Check sheet for the modelled part. Datum: model origin and axes. Units: mm. Face numbers are marked on the shaded views. A direction names the side the tool comes from. Round coordinates to 2 decimals unless told otherwise and drop trailing zeros. Order: outer loops, then holes, each group sorted by start corner. A loop starts at its lowest first (then second) coordinate and runs counter-clockwise, first axis right, second up. Notation, with made-up numbers: (80, -40) -> (90, -40) arc R13 cw to (90, -28) -> close; hole circle Ø4 at (61.5, 51). An arc over 180 degrees is marked (long way). Answer in a Markdown table with one row per item.
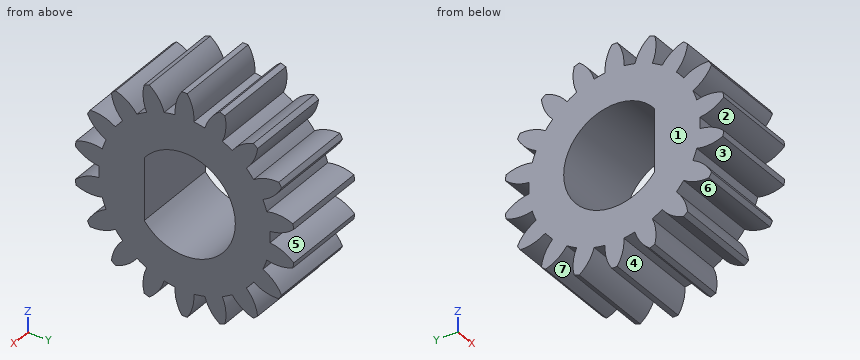
from build123d import *

# Parameters (mm, degrees)
BASPROSKE_W     = 4
BASPROSKE_H     = 5
TOOTHCUT_DEPTH  = 9.124038405
TEETHCUTS_COUNT = 18
TEETHCUTS_ANGLE = 340
BORE_DEPTH      = 50.0000508


with BuildPart() as part:
    # BasProSke → Base-Revolve (revolve)
    with BuildSketch(Plane(origin=(0, 0, 0), x_dir=(1, 0, 0), z_dir=(0, 1, 0)), mode=Mode.PRIVATE) as base_revolve_sk:
        with Locations((2, 2.5)):
            Rectangle(BASPROSKE_W, BASPROSKE_H)
    revolve(base_revolve_sk.sketch.rotate(Axis((-10, 0, 0), (1, 0, 0)), 180), axis=Axis((-10, 0, 0), (1, 0, 0)))

    # TooCutSke → ToothCut (cut, through all)
    with BuildSketch(Plane(origin=(0, 0, 0), x_dir=(0, 0, -1), z_dir=(1, 0, 0))):
        with BuildLine():
            ThreePointArc((0.25527463, 3.865580275), (0, 3.874), (-0.25527463, 3.865580275))
            ThreePointArc((-0.25527463, 3.865580275), (-0.416281865, 4.46052923), (-0.768562654, 4.96628197))
            ThreePointArc((-0.768562654, 4.96628197), (0, 5.0254), (0.768562654, 4.96628197))
            ThreePointArc((0.768562654, 4.96628197), (0.416281865, 4.46052923), (0.25527463, 3.865580275))
        make_face()
    toothcut = extrude(amount=TOOTHCUT_DEPTH, mode=Mode.SUBTRACT)

    # TeethCuts: ToothCut ×18 about axis
    teethcuts_axis = Axis((-10, 0, 0), (1, 0, 0))
    for i in range(1, TEETHCUTS_COUNT):
        add(toothcut.rotate(teethcuts_axis, i * TEETHCUTS_ANGLE / (TEETHCUTS_COUNT - 1)), mode=Mode.SUBTRACT)

    # BorSke → Bore (cut, symmetric)
    with BuildSketch(Plane(origin=(0, 0, 0), x_dir=(0, 0, -1), z_dir=(1, 0, 0))):
        with BuildLine():
            Line((-1.40479833, -1.82), (1.40479833, -1.82))
            ThreePointArc((1.40479833, -1.82), (0, 2.299099464), (-1.40479833, -1.82))
        make_face()
    extrude(amount=BORE_DEPTH, both=True, mode=Mode.SUBTRACT)


solid = part.part
Item 1: Cross-section at D-D (y = -2). Record the boundary of the cut face in (x, z).
Result sheet:
| item | result |
|---|---|
| outline | (0, -3.32) -> (4, -3.32) -> (4, 3.32) -> (0, 3.32) -> close |
Item 2: Set-up check for the marked faces 5, 6 and 7: record each of +Z, -Z, +X, -X, +Y, -Y from which the full face is reachable in a straight line by a thin tool's end or side.
Result sheet:
| item | result |
|---|---|
| face 5 | +X, -X, +Y |
| face 6 | +X, -X |
| face 7 | -Z, +X, -X |
Item 3: Cross-section at A-A (y = 0). Record the boundary of the cut face in (x, z).
Result sheet:
| item | result |
|---|---|
| outline | (0, -5) -> (4, -5) -> (4, -2.3) -> (0, -2.3) -> close; (0, 2.3) -> (4, 2.3) -> (4, 5) -> (0, 5) -> close |
Item 4: Cross-section at C-C (z = 4.5). Record the boundary of the cut face in (x, y).
Result sheet:
| item | result |
|---|---|
| outline | (0, -1.86) -> (4, -1.86) -> (4, -1.33) -> (0, -1.33) -> close; (0, -0.35) -> (4, -0.35) -> (4, 0.35) -> (0, 0.35) -> close; (0, 1.33) -> (4, 1.33) -> (4, 1.86) -> (0, 1.86) -> close |
Item 5: Cross-section at B-B (z = 0). Record the boundary of the cut face in (x, y).
Result sheet:
| item | result |
|---|---|
| outline | (0, -3.87) -> (4, -3.87) -> (4, -1.82) -> (0, -1.82) -> close; (0, 2.3) -> (4, 2.3) -> (4, 3.87) -> (0, 3.87) -> close |
Item 6: Depth check by flat-ended pin: P1, Ø2, axis at x = 1.5, y = 3.5, coming from the +Z side; P2, Ø2, axis at x = 2.5, y = 3, coming from the -Z side; P3, Ø2, axis at x = 2, y = -2.5, coming from the -Z side. Enter the tip coordinate at first touch or a pass-through.
Result sheet:
| item | result |
|---|---|
| P1 | stops at z = 3.91 |
| P2 | stops at z = -3.91 |
| P3 | stops at z = -4.74 |
Item 7: Mould release check, pull along Y, two halves, no side actions. Record for the marked faces 1, 2, 3 and 4: pulls with the +Y half, pulls with the -Y half, needs draft (parallel to the pull), parting line crosses it, or undercut.
Result sheet:
| item | result |
|---|---|
| face 1 | needs draft |
| face 2 | pulls with the -Y half |
| face 3 | undercut |
| face 4 | undercut |
Item 8: Scan lines: line 1 (Z direction, x = 0.3, y = -3.75); line 2 (Y direction, x = 1.1, z = 0); line 3 (Y direction, x = 0.6, z = -3.5). Record each from-to range of solid material in increasing order. Write a range as [from, to].
Result sheet:
| item | result |
|---|---|
| line 1 | z = [-2.56, -1.68], [-1.09, 1.09], [1.68, 2.56] |
| line 2 | y = [-3.87, -1.82], [2.3, 3.87] |
| line 3 | y = [-3.26, -2.4], [-1.72, 1.72], [2.4, 3.26] |
